from build123d import *

# Parameters (mm, degrees)
SM_BASE_FLANGE_1_DEPTH = 50
OTHER_START            = -40.658639918
OTHER_1_OUTLINE_W      = 38
OTHER_1_OUTLINE_H      = 8
OTHER_1_DEPTH          = 3.535533906
OTHER_START_2          = -76.013978978
OTHER_1_2_OUTLINE_W    = 10
OTHER_1_2_OUTLINE_H    = 8
OTHER_1_2_DEPTH        = 3.535533906
OTHER_1_3_OUTLINE_W    = 7
OTHER_1_3_OUTLINE_H    = 10
OTHER_1_3_DEPTH        = 3.535533906
OTHER_START_3          = -35.355339059
OTHER_1_4_OUTLINE_W    = 7
OTHER_1_4_OUTLINE_H    = 38
OTHER_1_4_DEPTH        = 3.535533906
CUT_EXTRUDE_3_DEPTH    = 10
CUT_EXTRUDE_4_DEPTH    = 10


# Read off the part's stored shape, not the designer's step: Затупленный угол1
# Sheet-metal steps are written as plain solids
with BuildPart() as part:
    # Sketch 1 → Базовая кромка1 (new body)
    with BuildSketch(Plane.XY):
        with BuildLine():
            Line((0, 0), (0, 54.804758849))
            ThreePointArc((0, 54.804758849), (0.489581401, 58.605778722), (1.926366943, 62.158677443))
            Line((1.926366943, 62.158677443), (21.215755371, 96.450923538))
            ThreePointArc((21.215755371, 96.450923538), (22.1736124, 98.819522686), (22.5, 101.353535934))
            Line((22.5, 101.353535934), (22.5, 108.7340251))
            ThreePointArc((22.5, 108.7340251), (19.571067812, 115.805092912), (12.5, 118.7340251))
            Line((12.5, 118.7340251), (-57.5, 118.7340251))
            Line((-57.5, 118.7340251), (-57.5, 123.7340251))
            Line((-57.5, 123.7340251), (12.5, 123.7340251))
            ThreePointArc((12.5, 123.7340251), (23.106601718, 119.340626818), (27.5, 108.7340251))
            Line((27.5, 108.7340251), (27.5, 101.353535934))
            ThreePointArc((27.5, 101.353535934), (27.010418599, 97.552516061), (25.573633057, 93.99961734))
            Line((25.573633057, 93.99961734), (6.284244629, 59.707371245))
            ThreePointArc((6.284244629, 59.707371245), (5.3263876, 57.338772097), (5, 54.804758849))
            Line((5, 54.804758849), (5, 0))
            Line((5, 0), (0, 0))
        make_face()
    extrude(amount=SM_BASE_FLANGE_1_DEPTH)

    # Other 1 outline → Other 1 (cut)
    with BuildSketch(Plane(origin=(0, 0, 0), x_dir=(0.7071067811865474, 0, -0.7071067811865477), z_dir=(0.7071067811865476, 0, 0.7071067811865476)).offset(OTHER_START)):
        with Locations((-55, 121)):
            Rectangle(OTHER_1_OUTLINE_W, OTHER_1_OUTLINE_H)
    extrude(amount=OTHER_1_DEPTH, mode=Mode.SUBTRACT)

    # Other 1 2 outline → Other 1 2 (cut)
    with BuildSketch(Plane(origin=(0, 0, 0), x_dir=(0.7071067811865474, 0, 0.7071067811865477), z_dir=(0.7071067811865476, 0, -0.7071067811865476)).offset(OTHER_START_2)):
        with Locations((-5, -121)):
            Rectangle(OTHER_1_2_OUTLINE_W, OTHER_1_2_OUTLINE_H)
    extrude(amount=OTHER_1_2_DEPTH, mode=Mode.SUBTRACT)

    # Other 1 3 outline → Other 1 3 (cut)
    with BuildSketch(Plane(origin=(0, 0, 0), x_dir=(1, 0, 0), z_dir=(0, 0.7071067811865476, 0.7071067811865476))):
        with Locations((2.5, 0)):
            Rectangle(OTHER_1_3_OUTLINE_W, OTHER_1_3_OUTLINE_H)
    extrude(amount=OTHER_1_3_DEPTH, mode=Mode.SUBTRACT)

    # Other 1 4 outline → Other 1 4 (cut)
    with BuildSketch(Plane(origin=(0, 0, 0), x_dir=(1, 0, 0), z_dir=(0, 0.7071067811865476, -0.7071067811865476)).offset(OTHER_START_3)):
        with Locations((2.5, -21)):
            Rectangle(OTHER_1_4_OUTLINE_W, OTHER_1_4_OUTLINE_H)
    extrude(amount=OTHER_1_4_DEPTH, mode=Mode.SUBTRACT)

    # Эскиз4 → Вырез-Вытянуть3 (cut)
    with BuildSketch(Plane.XZ.offset(-118.7340251)):
        with BuildLine():
            Line((-35, 18.5), (-42, 18.5))
            ThreePointArc((-42, 18.5), (-48.5, 25), (-42, 31.5))
            Line((-42, 31.5), (-35, 31.5))
            ThreePointArc((-35, 31.5), (-28.5, 25), (-35, 18.5))
        make_face()
        with BuildLine():
            Line((-3, 18.5), (-10, 18.5))
            ThreePointArc((-10, 18.5), (-16.5, 25), (-10, 31.5))
            Line((-10, 31.5), (-3, 31.5))
            ThreePointArc((-3, 31.5), (3.5, 25), (-3, 18.5))
        make_face()
    extrude(amount=-CUT_EXTRUDE_3_DEPTH, mode=Mode.SUBTRACT)

    # Эскиз5 → Вырез-Вытянуть4 (cut)
    with BuildSketch(Plane.ZY):
        with BuildLine():
            Line((18.5, 10.5), (18.5, 17.5))
            ThreePointArc((18.5, 17.5), (25, 24), (31.5, 17.5))
            Line((31.5, 17.5), (31.5, 10.5))
            ThreePointArc((31.5, 10.5), (25, 4), (18.5, 10.5))
        make_face()
        with BuildLine():
            Line((18.5, 35.5), (18.5, 42.5))
            ThreePointArc((18.5, 42.5), (25, 49), (31.5, 42.5))
            Line((31.5, 42.5), (31.5, 35.5))
            ThreePointArc((31.5, 35.5), (25, 29), (18.5, 35.5))
        make_face()
    extrude(amount=-CUT_EXTRUDE_4_DEPTH, mode=Mode.SUBTRACT)


solid = part.part
The listing builds one solid part. Answer for the finished solid, in the listing's coordinates (mm). A direction names the side the tool comes from. Give positions to 0.01 mm unless a question says otherwise; leave off trailing zeros. Write each loop counter-clockwise with the first axis right and the second up, starting at its lowest first coordinate (ties: lowest second). Pieces come first, ordered by that corner, then holes.
Item 1: Section B-B, the plane x = -45 is taken. Write down the section's boundary in (y, z).
Item 2: Section C-C, the plane z = 39 is taken. Write down the section's boundary in (x, y), plus the area to 3 significant figures.
Item 3: Flat-ended cylindrical pins translate along their axes: P1, Ø25, axis at x = -14, z = 28, coming from the -Y side; P2, Ø4, axis at y = 75.5, z = 40.5, coming from the +X side; P3, Ø12, axis at y = 44.5, z = 13, coming from the +X side; P4, Ø5, axis at y = 110, z = 28, coming from the +X side. Find the tip coordinate at first contact, or state that the pin passes through.
Item 4: Determine the mould class of faces 5 (the flat face through (-55, 121.3, 2.5)), 6 (the cylindrical face through (-28.5, 121.2, 25.1)), 7 (the cylindrical face through (19.648, 115.727, 24.65)) for opening direction Z: released by +Z, released by -Z, zero draft, split by the parting line, or undercut.
Item 5: Section D-D, the plane y = 19 is taken. Write down the section's boundary in (x, z), plus the area to 3 significant figures.
Item 6: Section A-A, the plane z = 25 is taken. Count the separate pieces of the cut face and the enclosed holes in it, plus the area to 3 significant figures.
Item 7: Which of the six approach directions +Z, -Z, +X, -X, +Y, -Y give full straight-line access (tool end or side, diameter ignored) to faces 1 (the flat face through (-57.5, 121, 25)), 2 (the cylindrical face through (3.5, 121.2, 25.1)), 3 (the cylindrical face through (2, 4, 25)), 4 (the flat face through (-7, 121, 31.5))?
Item 8: Find the intervals of material crossed by line 1 along X through (y, z) = (41.5, 34.5); line 2 along X through (y, z) = (119.5, 24); line 3 along Y through (x, z) = (-40, 13), in increasing order.
Completed:
1. outline: (118.73, 0) - (123.73, 0) - (123.73, 19.23) - (118.73, 19.23) - close; (118.73, 30.77) - (123.73, 30.77) - (123.73, 50) - (118.73, 50) - close
2. outline: (-57.5, 118.73) - (12.5, 118.73) arc R10 cw to (22.5, 108.73) - (22.5, 101.35) arc R10 cw to (21.22, 96.45) - (1.93, 62.16) arc R15 ccw to (0, 54.8) - (0, 0) - (5, 0) - (5, 54.8) arc R10 cw to (6.28, 59.71) - (25.57, 94) arc R15 ccw to (27.5, 101.35) - (27.5, 108.73) arc R15 ccw to (12.5, 123.73) - (-57.5, 123.73) - close
2. area: 1,020 mm2
3. P1: stops at y = 118.73
3. P2: stops at x = 16.29
3. P3: stops at x = 5
3. P4: stops at x = 27.5
4. face 5: released by -Z
4. face 6: undercut
4. face 7: zero draft
5. outline: (0, 0) - (5, 0) - (5, 18.68) - (0, 18.68) - close; (0, 31.32) - (5, 31.32) - (5, 50) - (0, 50) - close
5. area: 187 mm2
6. separate pieces: 5
6. enclosed holes: 0
6. area: 620 mm2
7. face 1: +Z, -Z, -X, +Y, -Y
7. face 2: +Y
7. face 3: +X, -X
7. face 4: +Y, -Y
8. line 1: x = 0 to 5
8. line 2: x = -57.5 to -48.42, -28.58 to -16.42, 3.42 to 22.94
8. line 3: y = 118.73 to 123.73
